Autodesk Inventor part; units mm, degrees
ref_plane "Work Plane2" through (-20.1778, -24.509, -31.7) normal (0, 0, -1) x (0, 1, 0)
ref_plane "Work Plane4" through (-15.4903, -24.384, -27.0904) normal (0, 0, 1) x (1, 0, 0)
ref_plane "Work Plane5" through (-21.5003, -26, -22.155) normal (0, 1, 0) x (0, 0, 1)
ref_plane "Work Plane1" through (0, 0, 0) normal (0, 0, 1) x (1, 0, 0)
sketch "Sketch1" plane through (0, 0, 0) normal (0, 0, 1) x (1, 0, 0)
  line L0 (-18.6403, -24.384) -> (-6.5903, -24.384)
  line L1 (-6.5903, -24.384) -> (-6.5903, -23.384)
  line L2 (-6.5903, -23.384) -> (-18.6403, -23.384)
  line L3 (-18.6403, -23.384) -> (-18.6403, -24.384)
  line L4 (-18.4403, -23.584) -> (-6.7903, -23.584)
  line L5 (-6.7903, -23.584) -> (-6.7903, -24.184)
  line L6 (-6.7903, -24.184) -> (-18.4403, -24.184)
  line L7 (-18.4403, -24.184) -> (-18.4403, -23.584)
  point P0 (0, 0)
  dimension "d0" = 0.2
ref_plane "Work Plane2" through (-20.1778, -24.509, -31.7) normal (0, 0, -1) x (0, 1, 0)
extrude "Extrusion1" add sketch "Sketch1" against normal up to surface (31.7 mm away) contours L4 L5 L6 L7
sketch "Sketch2" plane through (-18.4403, -24.184, 0) normal (0, -1, 0) x (1, 0, 0)
  line L0 (12.815, -1.2) -> (-1.155, -1.2)
  line L1 (-1.155, -22.155) -> (12.815, -22.155)
  line L2 (12.815, -2) -> (-1.155, -2)
  line L3 (-1.155, -21.355) -> (12.815, -21.355)
  line L4 (0, 0) -> (0, -31.7)
  line L5 (11.65, 0) -> (11.65, -31.7)
  point P0 (18.4403, 0)
  point P1 (11.65, -21.355)
  point P2 (11.65, -2)
  point P3 (0, -2)
  point P4 (0, -21.355)
  dimension "d3" = 0.8
  dimension "d4" = 0.8
ref_plane "Work Plane3" through (-12.6103, -25.6952, -11.6775) normal (0, 1, 0) x (0, 0, 1)
extrude "Extrusion2" add sketch "Sketch2" along normal up to surface (1.5112 mm away) contours L5 L3 L4 L2
sketch "Sketch3" plane through (-6.7903, -24.184, -21.355) normal (0, 0, -1) x (-1, 0, 0)
  line L0 (0, 0) -> (11.65, 0)
  line L1 (11.65, -1.5112) -> (0, -1.5112)
  line L2 (1, 0) -> (10.65, 0)
  line L3 (10.65, 0) -> (10.65, -1.5112)
  line L4 (10.65, -1.5112) -> (1, -1.5112)
  line L5 (1, -1.5112) -> (1, 0)
  line L6 (-1.05, -0.2) -> (2.45, -3.7)
  line L7 (8.7, -4.2) -> (12.7, -0.2)
  line L8 (0, 0) -> (0, -1.5112)
  line L9 (11.65, 0) -> (11.65, -1.5112)
  point P0 (-6.7903, 24.184)
  point P1 (1, -1.5112)
  dimension "d7" = 1
  dimension "d8" = 1
ref_plane "Work Plane4" through (-15.4903, -24.384, -27.0904) normal (0, 0, 1) x (1, 0, 0)
extrude "Extrusion3" add sketch "Sketch3" along normal up to surface (5.7354 mm away) contours L0 L3 L1 L5
sketch "Sketch4" plane through (-18.4403, -25.6952, -2) normal (0, -1, 0) x (1, 0, 0)
  line L0 (0, 2) -> (0, -29.7)
  line L1 (11.65, 2) -> (11.65, -29.7)
  line L2 (0, -14.85) -> (11.65, -14.85)
  line L3 (11.65, -14.85) -> (11.65, -13.85)
  line L4 (11.65, -13.85) -> (0, -13.85)
  line L5 (0, -13.85) -> (0, -14.85)
  line L6 (0, -5.2891) -> (11.65, -5.2891)
  line L7 (11.65, -5.2891) -> (11.65, -4.2891)
  line L8 (11.65, -4.2891) -> (0, -4.2891)
  line L9 (0, -4.2891) -> (0, -5.2891)
  point P0 (18.4403, 2)
  point P1 (0, -4.2891)
  point P2 (0, -5.2891)
  point P3 (0, -13.85)
  dimension "d11" = 1
  dimension "d12" = 1
ref_plane "Work Plane5" through (-21.5003, -26, -22.155) normal (0, 1, 0) x (0, 0, 1)
extrude "Extrusion4" [suppressed]
fillet "Fillet1" [suppressed]
equation "\"d8\" = d7"
equation "\"d12\" = d11"
properties part number "MCU seatbelt"
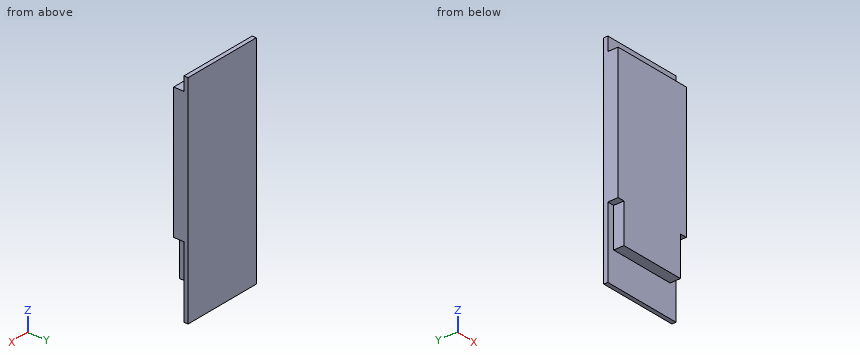
Read the model definition and answer for the solid it produces. Units are mm, in the model's axes. Coordinates: 2 decimals unless noted, no trailing zeros. Write each loop counter-clockwise with the first axis right and the second up, starting at its lowest first coordinate (ties: lowest second). Pieces come first, ordered by that corner, then holes. Notation, with made-up numbers: M -4,-19.75 L 32,-19.75 A26 cw 32,14.25 Z; hole C 32,76.25 d11. An arc over 180 degrees is marked long. Use a Markdown table: item, result.
Q1. Straight lines are drawn through the part: L1, parallel to Z at x = -10.5, y = -25.05; L2, parallel to Y at x = -17, z = -30; L3, parallel to Z at x = -17.5, y = -24.65 (3 decimals). For each, find the intervals that lie inside material, in ascending order. Write a range as [from, to].
Answer block:
| item | result |
|---|---|
| L1 | z = [-27.09, -2] |
| L2 | y = [-24.18, -23.58] |
| L3 | z = [-21.355, -2] |
Q2. Each of these flat-tipped pins is pushed along its axis until it touches: pin 1 Ø0.6 at (x, z) = (-13.5, -1.5) entering from -Y; pin 2 Ø0.8 at (x, y) = (-13.5, -25) entering from -Z; pin 3 Ø0.5 at (x, y) = (-12, -25) entering from +Z. Where does it stop, or does it pass through?
Answer block:
| item | result |
|---|---|
| pin 1 | stops at y = -24.18 |
| pin 2 | stops at z = -27.09 |
| pin 3 | stops at z = -2 |
Q3. The part is cut by section A-A, the plane x = -16.5. Write down the section's boundary in (y, z), then the cut area to 3 significant figures.
Answer block:
| item | result |
|---|---|
| outline | M -25.7,-27.09 L -24.18,-27.09 L -24.18,-31.7 L -23.58,-31.7 L -23.58,0 L -24.18,0 L -24.18,-2 L -25.7,-2 Z |
| area | 56.9 mm2 |
Q4. The part is cut by section B-B, the plane y = -24.75. Write down the section's boundary in (x, z) (3 decimals), then the cut area to 3 significant figures.
Answer block:
| item | result |
|---|---|
| outline | M -18.44,-21.355 L -17.44,-21.355 L -17.44,-27.09 L -7.79,-27.09 L -7.79,-21.355 L -6.79,-21.355 L -6.79,-2 L -18.44,-2 Z |
| area | 281 mm2 |
